```python
from build123d import *

# Parameters (mm, degrees)
SKETCH1_R              = 2.925
SKETCH1_R_2            = 1.75
MIDDLE_RING_DEPTH      = 0.8
SKETCH2_R              = 2.35
SKETCH2_R_2            = 1.75
OUTER_BODY_DEPTH       = 7.35
SKETCH3_R              = 2.625
SKETCH3_R_2            = 1.75
OUTER_RIM_DEPTH        = 0.5
MIDDLE_SLOT_DEPTH      = 9.873204044
MIDDLE_SLOT_DEPTH_BACK = 9.873204044
SIDE_SLOTS_DEPTH       = 9.859105574
SIDE_SLOTS_DEPTH_BACK  = 9.859105574
SKETCH7_W              = 1.8
SKETCH7_H              = 1.8
AXLE_CUT_DEPTH         = 7.9
BUSH_SLOT_DEPTH        = 17.691389996
BUSH_SLOT_DEPTH_BACK   = 17.691389996


with BuildPart() as part:
    # Sketch1 → Middle Ring (new, symmetric)
    with BuildSketch(Plane(origin=(0, 0, 0), x_dir=(0, 0, -1), z_dir=(1, 0, 0))):
        Circle(SKETCH1_R)
        Circle(SKETCH1_R_2, mode=Mode.SUBTRACT)
    extrude(amount=MIDDLE_RING_DEPTH, both=True)

    # Sketch2 → Outer Body (add, symmetric)
    with BuildSketch(Plane(origin=(0, 0, 0), x_dir=(0, 0, -1), z_dir=(1, 0, 0))):
        Circle(SKETCH2_R)
        Circle(SKETCH2_R_2, mode=Mode.SUBTRACT)
    extrude(amount=OUTER_BODY_DEPTH, both=True)

    # Sketch3 → Outer Rim (add)
    with BuildSketch(Plane(origin=(7.35, 0, 0), x_dir=(0, 0, -1), z_dir=(1, 0, 0))):
        Circle(SKETCH3_R)
        Circle(SKETCH3_R_2, mode=Mode.SUBTRACT)
    outer_rim = extrude(amount=OUTER_RIM_DEPTH)

    # Mirror1: Outer Rim across plane
    add(outer_rim.mirror(Plane(origin=(0, 0, 0), x_dir=(0, 0, 1), z_dir=(1, 0, 0))))

    # Sketch4 → Middle Slot (cut, two sides: drawn at the far end of the back side and taken through both)
    with BuildSketch(Plane.XY.offset(-MIDDLE_SLOT_DEPTH_BACK)):
        with BuildLine():
            Line((2.95, -0.5), (-2.95, -0.5))
            ThreePointArc((-2.95, -0.5), (-3.45, 0), (-2.95, 0.5))
            Line((-2.95, 0.5), (2.95, 0.5))
            ThreePointArc((2.95, 0.5), (3.45, 0), (2.95, -0.5))
        make_face()
        with BuildLine():
            Line((-10.8, 0.5), (-4.9, 0.5))
            ThreePointArc((-4.9, 0.5), (-4.4, 0), (-4.9, -0.5))
            Line((-4.9, -0.5), (-10.8, -0.5))
            ThreePointArc((-10.8, -0.5), (-11.3, 0), (-10.8, 0.5))
        make_face()
    extrude(amount=MIDDLE_SLOT_DEPTH + MIDDLE_SLOT_DEPTH_BACK, mode=Mode.SUBTRACT)

    # Sketch5 → Side Slots (cut, two sides: drawn at the far end of the back side and taken through both)
    with BuildSketch(Plane(origin=(0, 0, 0), x_dir=(1, 0, 0), z_dir=(0, 1, 0)).offset(-SIDE_SLOTS_DEPTH_BACK)):
        with BuildLine():
            Line((10.95, -0.5), (4.75, -0.5))
            ThreePointArc((4.75, -0.5), (4.25, 0), (4.75, 0.5))
            Line((4.75, 0.5), (10.95, 0.5))
            ThreePointArc((10.95, 0.5), (11.45, 0), (10.95, -0.5))
        make_face()
    extrude(amount=SIDE_SLOTS_DEPTH + SIDE_SLOTS_DEPTH_BACK, mode=Mode.SUBTRACT)

    # Sketch6 → Large Bush (revolve)
    with BuildSketch(Plane.XY, mode=Mode.PRIVATE) as large_bush_sk:
        Polygon((-15.85, 0), (-15.85, 3.7), (-14.45, 3.7), (-14.45, 2.85), (-9.35, 2.85), (-9.35, 3.7), (-7.95, 3.7), (-7.95, 2.95), (-7.15, 2.95), (-7.15, 0), align=None)
    revolve(large_bush_sk.sketch.rotate(Axis((0, 0, 0), (-1, 0, 0)), 257.715539925), axis=Axis((0, 0, 0), (-1, 0, 0)))

    # Sketch7 → Axle Cut (cut)
    with BuildSketch(Plane.ZY.offset(15.85)):
        with BuildLine():
            Line((-0.9, 0.9), (0.9, 0.9))
            Line((0.9, 0.9), (0.9, 2.224859546))
            ThreePointArc((0.9, 2.224859546), (0.45844143, 2.355808026), (0, 2.4))
            ThreePointArc((0, 2.4), (-0.45844143, 2.355808026), (-0.9, 2.224859546))
            Line((-0.9, 2.224859546), (-0.9, 0.9))
        make_face()
        Rectangle(SKETCH7_W, SKETCH7_H)
        with BuildLine():
            Line((-2.224859546, -0.9), (-0.9, -0.9))
            Line((-0.9, -0.9), (-0.9, 0.9))
            Line((-0.9, 0.9), (-2.224859546, 0.9))
            ThreePointArc((-2.224859546, 0.9), (-2.355808026, 0.458441427), (-2.4, -5e-09))
            ThreePointArc((-2.4, -5e-09), (-2.355808026, -0.458441432), (-2.224859546, -0.9))
        make_face()
        with BuildLine():
            Line((0.9, 0.9), (0.9, -0.9))
            Line((0.9, -0.9), (2.224859546, -0.9))
            ThreePointArc((2.224859546, -0.9), (2.355808026, -0.45844143), (2.4, 0))
            ThreePointArc((2.4, 0), (2.355808026, 0.45844143), (2.224859546, 0.9))
            Line((2.224859546, 0.9), (0.9, 0.9))
        make_face()
        with BuildLine():
            ThreePointArc((-0.9, -2.224859546), (-0.45844143, -2.355808026), (0, -2.4))
            ThreePointArc((0, -2.4), (0.45844143, -2.355808026), (0.9, -2.224859546))
            Line((0.9, -2.224859546), (0.9, -0.9))
            Line((0.9, -0.9), (-0.9, -0.9))
            Line((-0.9, -0.9), (-0.9, -2.224859546))
        make_face()
    extrude(amount=-AXLE_CUT_DEPTH, mode=Mode.SUBTRACT)

    # Sketch9 → Bush Slot (cut, two sides: drawn at the far end of the back side and taken through both)
    with BuildSketch(Plane.XY.offset(-BUSH_SLOT_DEPTH_BACK)):
        with BuildLine():
            Line((-13.8, 0.5), (-10, 0.5))
            ThreePointArc((-10, 0.5), (-9.5, 0), (-10, -0.5))
            Line((-10, -0.5), (-13.8, -0.5))
            ThreePointArc((-13.8, -0.5), (-14.3, 0), (-13.8, 0.5))
        make_face()
    extrude(amount=BUSH_SLOT_DEPTH + BUSH_SLOT_DEPTH_BACK, mode=Mode.SUBTRACT)


solid = part.part
```
The listing builds one solid part. Answer for the finished solid, in the listing's coordinates (mm). A direction names the side the tool comes from. Coordinates: 2 decimals unless noted, no trailing zeros. Write each loop counter-clockwise with the first axis right and the second up, starting at its lowest first coordinate (ties: lowest second). Pieces come first, ordered by that corner, then holes. Notation, with made-up numbers: (24.5, -22) - (77.5, -22) arc R28 ccw to (77.5, 17) - close; hole circle Ø9 at (55.5, 70.25). An arc over 180 degrees is marked (long way). Return JSON: item names as keys, results as strings. Group by question number.
Q1. For a pull along Z with two mould halves and no side action, classify faces 4 (the flat face through (-12, 0.9, -2)), 5 (the cylindrical face through (-11.864, 0.728, -2.755)), 6 (the flat face through (-15.85, -1.4, -1.1)) as +Z half, -Z half, draft (parallel to the pull), parting line (faces both ways), or undercut.
Q2. Flat-ended cylindrical pins translate along their axes: pin 1 Ø1 at (x, y) = (-8, -1) entering from -Z; pin 2 Ø0.7 at (x, z) = (-5.5, 2) entering from -Y; pin 3 Ø1.1 at (y, z) = (0, -1.5) entering from -X; pin 4 Ø2.5 at (y, z) = (0, 1) entering from -X. Find the tip coordinate at first contact, or state that the pin passes through.
Q3. The part is cut by section A-A on x = -10.5. Write down the section's boundary in (y, z), and give its area (3 significant figures).
Q4. Find the intervals of material crossed by line 1 along X through (y, z) = (-3.25, 1.25); line 2 along Y through (x, z) = (-4, 0), in increasing order. Write a range as [from, to].
Q5. Which of the six approach directions +Z, -Z, +X, -X, +Y, -Y give full straight-line access (tool end or side, diameter ignored) to faces 1 (the flat face through (0, -0.5, 2)), 2 (the flat face through (0.8, -2.5, -0.2)), 3 (the flat face through (6, -2, 0.5))?
Q6. The part is cut by section B-B on y = 0.25. State how many separate pieces and enclosed holes the cut face has, and give its area (3 significant figures).
Evaluation:
{
 "1": {"face 4": "undercut", "face 5": "parting line", "face 6": "draft"},
 "2": {"pin 1": "stops at z = -3.67", "pin 2": "stops at y = -1.67", "pin 3": "stops at x = -7.95", "pin 4": "stops at x = -15.85"},
 "3": {"outline": "(-2.22, -0.9) arc R2.4 cw to (-2.22, 0.9) - (-0.9, 0.9) - (-0.9, 2.22) arc R2.4 cw to (-0.5, 2.35) - (-0.5, 2.81) arc R2.85 ccw to (-0.5, -2.81) - (-0.5, -2.35) arc R2.4 cw to (-0.9, -2.22) - (-0.9, -0.9) - close; (0.5, -2.81) arc R2.85 ccw to (0.5, 2.81) - (0.5, 2.35) arc R2.4 cw to (0.9, 2.22) - (0.9, 0.9) - (2.22, 0.9) arc R2.4 cw to (2.22, -0.9) - (0.9, -0.9) - (0.9, -2.22) arc R2.4 cw to (0.5, -2.35) - close", "area": "11.0 mm2"},
 "4": {"line 1": "x = [-15.85, -14.45], [-9.35, -7.95]", "line 2": "y = [-2.35, -1.75], [1.75, 2.35]"},
 "5": {"face 1": "+Z, -Z", "face 2": "-Y", "face 3": "+X, +Y, -Y"},
 "6": {"separate pieces": "7", "enclosed holes": "0", "area": "19.4 mm2"}
}
